Autodesk Inventor part; units mm, degrees
ref_plane "YZ Plane" through (0, 0, 0) normal (1, 0, 0) x (0, 1, 0)
ref_plane "XZ Plane" through (0, 0, 0) normal (0, 1, 0) x (-1, 0, 0)
ref_plane "XY Plane" through (0, 0, 0) normal (0, 0, 1) x (1, 0, 0)
sketch "Sketch1" plane through (0, 0, 0) normal (0, 1, 0) x (-1, 0, 0)
  line L0 (0, 0) -> (20, 0)
  line L1 (20, 0) -> (20, -190)
  line L2 (20, -190) -> (0, -190)
  line L3 (0, -190) -> (0, 0)
  dimension "d0" = 20
  dimension "d1" = 190
extrude "Extrusion1" add sketch "Sketch1" along normal blind 1.5
sketch "Sketch2" plane through (0, 0, 0) normal (0, -1, 0) x (1, 0, 0)
  line L0 (0, 0) -> (-1.5, 0)
  line L1 (-1.5, 0) -> (-1.5, -190)
  line L2 (-1.5, -190) -> (0, -190)
  line L3 (0, -190) -> (0, 0)
  dimension "d4" = 1.5
  dimension "d5" = 190
extrude "Extrusion2" add sketch "Sketch2" against normal blind 10
sketch "Sketch3" plane through (0, 1.5, 0) normal (0, 1, 0) x (1, 0, 0)
  line L0 (-20, 0) -> (-1.5, 0)
  line L1 (-20, 0) -> (-1.5, 0)
  line L2 (-1.5, 0) -> (-1.5, 18.5)
  line L3 (-1.5, 18.5) -> (-20, 18.5)
  line L4 (-20, 18.5) -> (-20, 0)
  line L5 (-20, 190) -> (-1.5, 190)
  line L6 (-1.5, 190) -> (-1.5, 171.5)
  line L7 (-1.5, 171.5) -> (-20, 171.5)
  line L8 (-20, 171.5) -> (-20, 190)
  line L9 (-20, 171.5) -> (-13, 171.5)
  line L10 (-13, 171.5) -> (-13, 178.5)
  line L11 (-13, 178.5) -> (-20, 178.5)
  line L12 (-20, 178.5) -> (-20, 171.5)
  line L13 (-20, 171.5) -> (-6, 171.5)
  line L14 (-6, 171.5) -> (-6, 185.5)
  line L15 (-6, 185.5) -> (-20, 185.5)
  line L16 (-20, 185.5) -> (-20, 171.5)
  circle A0 centre (-6, 185.5) radius 2
  circle A1 centre (-13, 178.5) radius 2
  line L17 (-20, 18.5) -> (-13, 18.5)
  line L18 (-13, 18.5) -> (-13, 11.5)
  line L19 (-13, 11.5) -> (-20, 11.5)
  line L20 (-20, 11.5) -> (-20, 18.5)
  line L21 (-20, 18.5) -> (-6, 18.5)
  line L22 (-6, 18.5) -> (-6, 4.5)
  line L23 (-6, 4.5) -> (-20, 4.5)
  line L24 (-20, 4.5) -> (-20, 18.5)
  circle A2 centre (-13, 11.5) radius 2
  circle A3 centre (-6, 4.5) radius 2
  line L25 (-20, 190) -> (-20, 140)
  line L26 (-20, 140) -> (-20, 50)
  line L27 (-20, 140) -> (-10, 140)
  line L28 (-10, 140) -> (-10, 50)
  line L29 (-10, 50) -> (-20, 50)
  line L30 (-20, 50) -> (-20, 140)
  circle A4 centre (-10, 140) radius 2
  circle A5 centre (-10, 50) radius 2
  point P0 (0, 0)
  dimension "d8" = 18.5
  dimension "d9" = 18.5
  dimension "d10" = 18.5
  dimension "d11" = 18.5
  dimension "d12" = 7
  dimension "d13" = 7
  dimension "d14" = 14
  dimension "d15" = 14
  dimension "d16" = 4
  dimension "d17" = 4
  dimension "d18" = 7
  dimension "d19" = 7
  dimension "d20" = 14
  dimension "d21" = 14
  dimension "d22" = 4
  dimension "d23" = 4
  dimension "d26" = 50
  dimension "d27" = 90
  dimension "d28" = 10
  dimension "d29" = 4
  dimension "d30" = 4
extrude "Extrusion3" cut sketch "Sketch3" against normal blind 10 contours A3 L22 L23 | L23 L22 A3 | A2 L18 L19 | L19 L18 A2 | A0 L14 L15 | L15 L14 A0 | A1 L10 L11 | L11 L10 A1 | A4 L28 L27 | L27 L28 A4 | A5 L28 L29 | L29 L28 A5
properties part number "aluminium_profile_1"
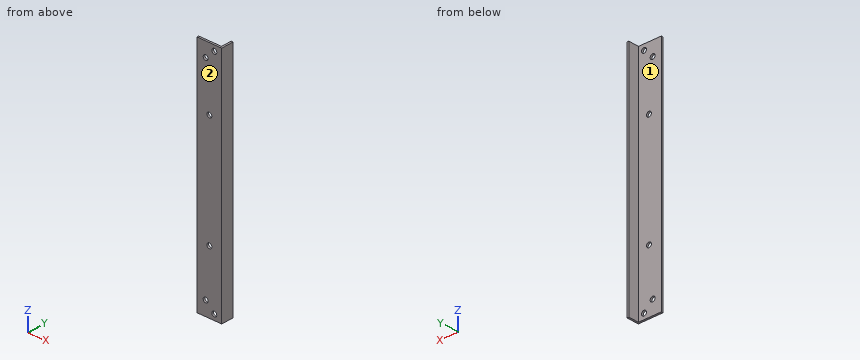
Check sheet for the modelled part. Datum: model origin and axes. Units: mm. Face numbers are marked on the shaded views. A direction names the side the tool comes from. Round coordinates to 2 decimals unless told otherwise and drop trailing zeros. Loops run counter-clockwise (first coordinate to the right, second up) from the corner with the lowest first, then second, coordinate; pieces in that order, holes last. Notation, with made-up numbers: M 46.5,-20 L 81.5,-20 A30 ccw 81.5,6 Z; hole C 79.5,-9 d7. An arc over 180 degrees is marked long. One line per question, with ' | ' between items. Start each with the question number.
Item 1: Gauge pin test, flat ends, axial feed: pin 1 Ø9 at (x, z) = (-10, -141.5) entering from +Y; pin 2 Ø1.5 at (y, z) = (3, -87) entering from -X. Record the tip position at first contact, or that the pin passes through.
Item 2: Section check B-B (z = -40). Record the boundary of the cut face in (x, y).
Item 3: Section check A-A (z = -140). Record the boundary of the cut face in (x, y).
Item 4: Section check C-C (x = -17.25). Record the boundary of the cut face in (y, z).
Item 5: Scan lines: probe 1 along Z at (x, y) = (-6, 0.3); probe 2 along Z at (x, y) = (-10, 1.15); probe 3 along X at (y, z) = (1.1, -140). Record each from-to range of solid material in increasing order.
Item 6: Set-up check for the marked faces 1 and 2: record each of +Z, -Z, +X, -X, +Y, -Y from which the full face is reachable in a straight line by a thin tool's end or side.
Item 7: Section check D-D (y = 8). Record the boundary of the cut face in (x, z), and give its area (3 significant figures).
Worked out:
1) pin 1: y = 1.5 | pin 2: x = -1.5
2) outline: M -20,0 L 0,0 L 0,10 L -1.5,10 L -1.5,1.5 L -20,1.5 Z
3) outline: M -20,0 L -12,0 L -12,1.5 L -20,1.5 Z; M -8,0 L 0,0 L 0,10 L -1.5,10 L -1.5,1.5 L -8,1.5 Z
4) outline: M 0,-190 L 1.5,-190 L 1.5,0 L 0,0 Z
5) probe 1: -190 to -187.5, -183.5 to -6.5, -2.5 to 0 | probe 2: -190 to -142, -138 to -52, -48 to 0 | probe 3: -20 to -12, -8 to 0
6) face 1: +Z, -Z, -X, +Y | face 2: +Z, -Z, +X, -X, -Y
7) outline: M -1.5,-190 L 0,-190 L 0,0 L -1.5,0 Z | area: 285 mm^2
